Geometry check sheet. Reference: drawing and pictorial views, mm from the part's lowest x, y, z. A direction names the side the tool comes from. Give positions to 0.01 mm unless a question says otherwise; leave off trailing zeros. Loops run counter-clockwise (first coordinate to the right, second up) from the corner with the lowest first, then second, coordinate; pieces in that order, holes last. Notation, with made-up numbers: (-24.5, -29.75) -> (31.5, -29.75) arc R16 cw to (31.5, -5.75) -> close; hole circle Ø11 at (-8.5, -25.75). An arc over 180 degrees is marked (long way). One line per item, written item: value. Start each with the question number.
(1) Sectioned sample at A-A, the plane x = 4.75. Record the cut outline in (y, z), then the cut area to 3 significant figures.
(2) Sectioned sample at B-B, the plane y = 6.25. Record the cut outline in (x, z) (1 decimal).
(3) Sectioned sample at C-C, the plane z = 4.75. Record the cut outline in (x, y).
(4) Gauge pin test, flat end, axial feed: pin 1 Ø5 at (x, z) = (27.47, 27.35) entering from +Y. Record the tip position at first contact, or that the pin passes through.
(5) Tool access check on the marked faces 1 and 2. Record the directions out of +Z, -Z, +X, -X, +Y, -Y that give a thin tool (end or side, any length) a straight path to the whole face; none if there is none.
(6) Sectioned sample at D-D, the plane x = 25.5. Record the cut outline in (y, z).
(7) Draft check along Z on the marked faces 3, 4 and 5. Enter one of: pulls with the +Z half, pulls with the -Z half, needs draft (parallel to the pull), parting line crosses it, or undercut.
(8) Scan lines: line 1 along Z through (x, y) = (35.25, 1.9); line 2 along X through (y, z) = (6.5, 11); line 3 along Z through (x, y) = (14, 6). Record each from-to range of solid material in increasing order. Write a range as from..to.
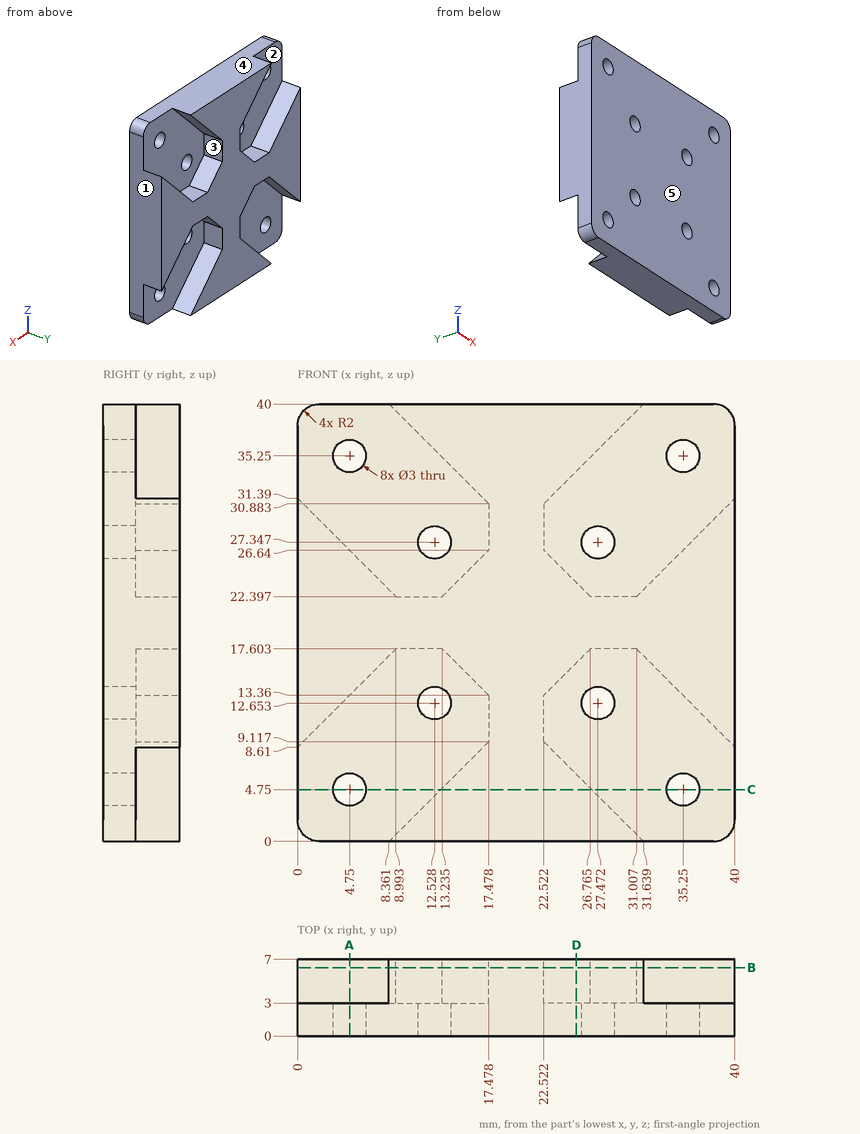
Calculated:
1. outline: (0, 0) -> (3, 0) -> (3, 3.25) -> (0, 3.25) -> close; (0, 6.25) -> (3, 6.25) -> (3, 13.36) -> (7, 13.36) -> (7, 26.64) -> (3, 26.64) -> (3, 33.75) -> (0, 33.75) -> close; (0, 36.75) -> (3, 36.75) -> (3, 40) -> (0, 40) -> close
1. area: 155 mm2
2. outline: (0, 8.6) -> (9, 17.6) -> (13.2, 17.6) -> (17.5, 13.4) -> (17.5, 9.1) -> (8.4, 0) -> (31.6, 0) -> (22.5, 9.1) -> (22.5, 13.4) -> (26.8, 17.6) -> (31, 17.6) -> (40, 8.6) -> (40, 31.4) -> (31, 22.4) -> (26.8, 22.4) -> (22.5, 26.6) -> (22.5, 30.9) -> (31.6, 40) -> (8.4, 40) -> (17.5, 30.9) -> (17.5, 26.6) -> (13.2, 22.4) -> (9, 22.4) -> (0, 31.4) -> close
3. outline: (0, 0) -> (3.25, 0) -> (3.25, 3) -> (0, 3) -> close; (6.25, 0) -> (33.75, 0) -> (33.75, 3) -> (26.89, 3) -> (26.89, 7) -> (13.11, 7) -> (13.11, 3) -> (6.25, 3) -> close; (36.75, 0) -> (40, 0) -> (40, 3) -> (36.75, 3) -> close
4. pin 1: stops at y = 3
5. face 1: +Z, -Z, +X, +Y, -Y
5. face 2: +Y
6. outline: (0, 0) -> (7, 0) -> (7, 6.14) -> (3, 6.14) -> (3, 16.34) -> (7, 16.34) -> (7, 23.66) -> (3, 23.66) -> (3, 33.86) -> (7, 33.86) -> (7, 40) -> (0, 40) -> close
7. face 3: undercut
7. face 4: pulls with the +Z half
7. face 5: needs draft
8. line 1: z = 0..3.25, 6.25..33.75, 36.75..40
8. line 2: x = 0..2.39, 17.48..22.52, 37.61..40
8. line 3: z = 0..5.64, 16.84..23.16, 34.36..40
